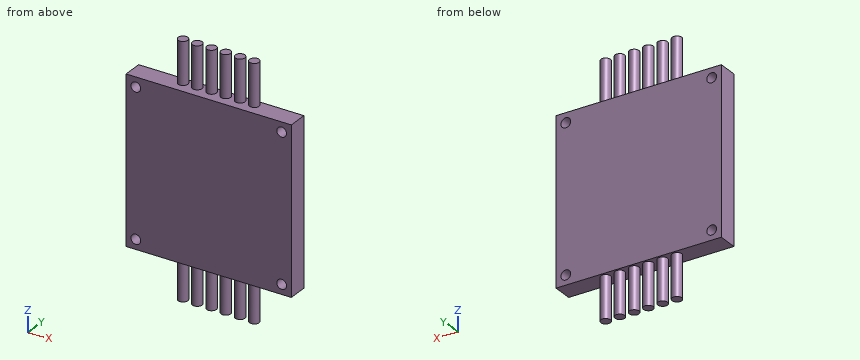
Autodesk Fusion 360 part; units mm, degrees
sketch "Sketch1" plane through (0, 0, 0) normal (0, 1, 0) x (1, 0, 0)
  line L0 (25.5, -25.5) -> (-25.5, -25.5)
  line L1 (-25.5, -25.5) -> (-25.5, 25.5)
  line L2 (-25.5, 25.5) -> (25.5, 25.5)
  line L3 (25.5, 25.5) -> (25.5, -25.5)
  line L4 (25.5, -25.5) -> (-25.5, 25.5) construction
  line L5 (-25.5, -25.5) -> (25.5, 25.5) construction
  circle A0 centre (-22.5, 22.5) radius 1.5
  circle A1 centre (22.5, 22.5) radius 1.5
  circle A2 centre (22.5, -22.5) radius 1.5
  circle A3 centre (-22.5, -22.5) radius 1.5
  dimension "d1" = 51
  dimension "d2" = 51
  dimension "d5" = 3
  dimension "d6" = 45
extrude "Extrude1" add sketch "Sketch1" along normal blind 6
sketch "Sketch2" plane through (0, 0, 25.5) normal (0, 0, 1) x (1, 0, 0)
  line L0 (-25.5, 0) -> (25.5, 0)
  line L1 (25.5, 0) -> (25.5, 6)
  line L2 (25.5, 6) -> (-25.5, 6)
  line L3 (-25.5, 6) -> (-25.5, 0)
  circle A0 centre (-10.5, 4) radius 1.5
  circle A1 centre (-6.1, 4) radius 1.5
  circle A2 centre (-1.7, 4) radius 1.5
  circle A3 centre (2.7, 4) radius 1.5
  circle A4 centre (7.1, 4) radius 1.5
  circle A5 centre (11.5, 4) radius 1.5
  dimension "d7" = 3
  dimension "d8" = 2
  dimension "d9" = 15
  dimension "d12" = -22
  dimension "d13" = 0
extrude "Extrude2" add sketch "Sketch2" along normal blind 13 contours A0 | A1 | A2 | A3 | A4 | A5
mirror "Mirror1" about plane through (0, 0, 0) normal (0, 0, 1) of "Extrude2"
Geometry check sheet. Reference: the model listing, model coordinates, mm. Round coordinates to 2 decimals unless told otherwise and drop trailing zeros. Order: outer loops, then holes, each group sorted by start corner. A loop starts at its lowest first (then second) coordinate and runs counter-clockwise, first axis right, second up. Notation, with made-up numbers: (27.25, 55.5) - (55.25, 55.5) arc R12 cw to (55.25, 59.5) - close; hole circle Ø8 at (16.5, 22.25). An arc over 180 degrees is marked (long way). Use a Markdown table: item, result. Add a question column.
1) Thickness scan on line 1 along Z through (x, y) = (22.5, 4); line 2 along Z through (x, y) = (8, 1.1). Record the ranges inside material, lowest first.
2) Section check B-B (z = -22.5). Record the cut outline in (x, y), then the cut area to 3 significant figures.
3) Section check D-D (x = -6.1). Record the cut outline in (y, z).
4) Section check A-A (x = -22.5). Record the cut outline in (y, z).
5) Section check C-C (y = 1.1). Record the cut outline in (x, z).
Established:
| question | item | result |
|---|---|---|
| 1 | line 1 | -25.5 to -24, -21 to 21, 24 to 25.5 |
| 1 | line 2 | -25.5 to 25.5 |
| 2 | outline | (-25.5, 0) - (-24, 0) - (-24, 6) - (-25.5, 6) - close; (-21, 0) - (21, 0) - (21, 6) - (-21, 6) - close; (24, 0) - (25.5, 0) - (25.5, 6) - (24, 6) - close |
| 2 | area | 270 mm2 |
| 3 | outline | (0, -25.5) - (2.5, -25.5) - (2.5, -38.5) - (5.5, -38.5) - (5.5, -25.5) - (6, -25.5) - (6, 25.5) - (5.5, 25.5) - (5.5, 38.5) - (2.5, 38.5) - (2.5, 25.5) - (0, 25.5) - close |
| 4 | outline | (0, -25.5) - (6, -25.5) - (6, -24) - (0, -24) - close; (0, -21) - (6, -21) - (6, 21) - (0, 21) - close; (0, 24) - (6, 24) - (6, 25.5) - (0, 25.5) - close |
| 5 | outline | (-25.5, -25.5) - (25.5, -25.5) - (25.5, 25.5) - (-25.5, 25.5) - close; hole circle Ø3 at (-22.5, -22.5); hole circle Ø3 at (-22.5, 22.5); hole circle Ø3 at (22.5, -22.5); hole circle Ø3 at (22.5, 22.5) |
